Study the drawing (mm; zero at the part's minimum x, y, z) and answer. Give positions to 0.01 mm unless a question says otherwise; leave off trailing zeros. Loops run counter-clockwise (first coordinate to the right, second up) from the corner with the lowest first, then second, coordinate; pieces in that order, holes last. Notation, with made-up numbers: (74.25, 28.5) - (86.25, 28.5) arc R17 ccw to (86.25, 61.5) - close; hole circle Ø3 at (72, 10). An arc over 180 degrees is marked (long way). Write item = value, one per line. Start each with the question number.
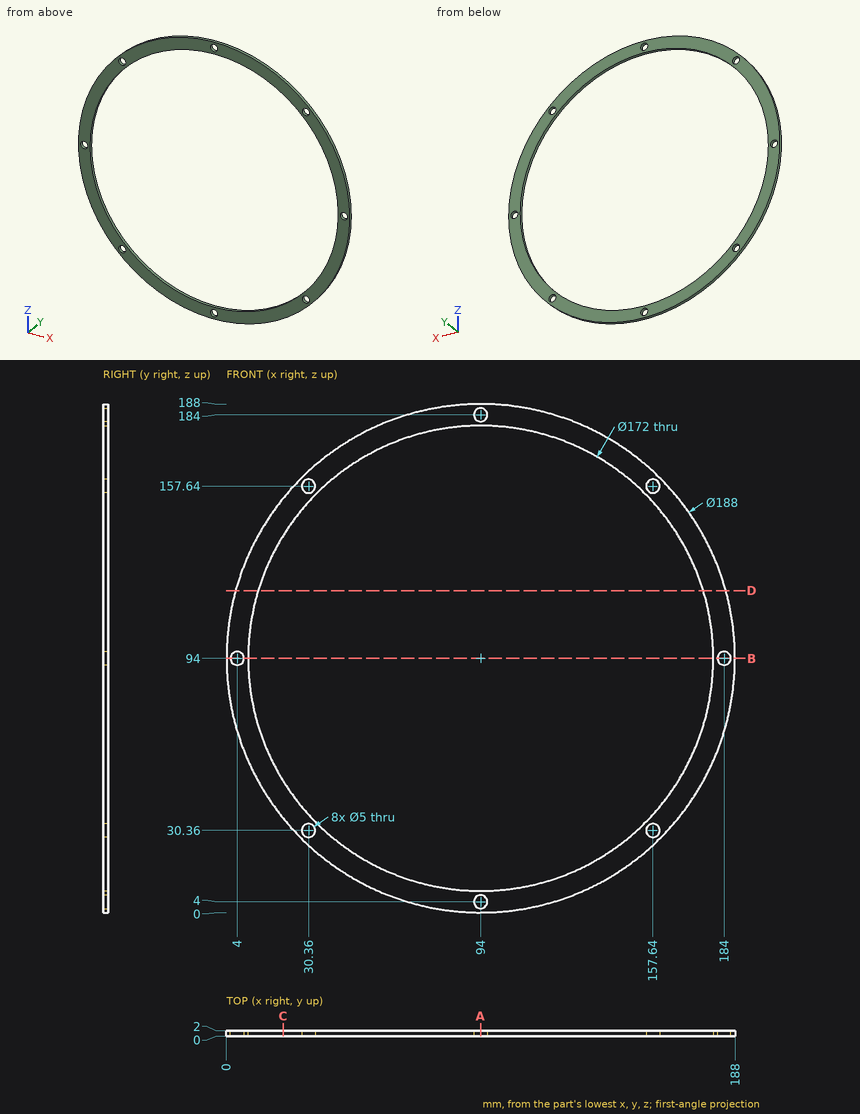
1. A cutting plane is placed at A-A on x = 94. Give the vertices of the cut face in (y, z), and give its area (3 significant figures).
2. A cutting plane is placed at C-C on x = 21. Give the vertices of the cut face in (y, z) (1 decimal).
3. A cutting plane is placed at B-B on z = 94. Give the vertices of the cut face in (x, y), and give its area (3 significant figures).
4. Given P1, Ø1, axis at y = 1.5, z = 77, coming from the -X side, flat-ended and moving along its own axis, determine where the tip first touches the part or whether it passes through.
5. A cutting plane is placed at D-D on z = 119. Give the vertices of the cut face in (x, y) (1 decimal), and give its area (3 significant figures).
6. Consider line 1 along X through (y, z) = (1.5, 29.5) (1 decimal); line 2 along X through (y, z) = (1.7, 32.5) (1 decimal); line 3 along X through (y, z) = (0.4, 74). Determine where each line is inside the solid, lowest interval first. Write a range as [from, to].
Reply:
q1.outline = (0, 0) - (2, 0) - (2, 1.5) - (0, 1.5) - close; (0, 6.5) - (2, 6.5) - (2, 8) - (0, 8) - close; (0, 180) - (2, 180) - (2, 181.5) - (0, 181.5) - close; (0, 186.5) - (2, 186.5) - (2, 188) - (0, 188) - close
q1.area = 12.0 mm^2
q2.outline = (0, 34.8) - (2, 34.8) - (2, 48.5) - (0, 48.5) - close; (0, 139.5) - (2, 139.5) - (2, 153.2) - (0, 153.2) - close
q3.outline = (0, 0) - (1.5, 0) - (1.5, 2) - (0, 2) - close; (6.5, 0) - (8, 0) - (8, 2) - (6.5, 2) - close; (180, 0) - (181.5, 0) - (181.5, 2) - (180, 2) - close; (186.5, 0) - (188, 0) - (188, 2) - (186.5, 2) - close
q3.area = 12.0 mm^2
q4.P1 = 1.46
q5.outline = (3.4, 0) - (11.7, 0) - (11.7, 2) - (3.4, 2) - close; (176.3, 0) - (184.6, 0) - (184.6, 2) - (176.3, 2) - close
q5.area = 33.3 mm^2
q6.line_1 = [25.6, 28], [32.7, 37.1], [150.9, 155.3], [160, 162.4]
q6.line_2 = [22.9, 29.1], [31.7, 33.9], [154.1, 156.3], [158.9, 165.1]
q6.line_3 = [2.15, 10.36], [177.64, 185.85]
